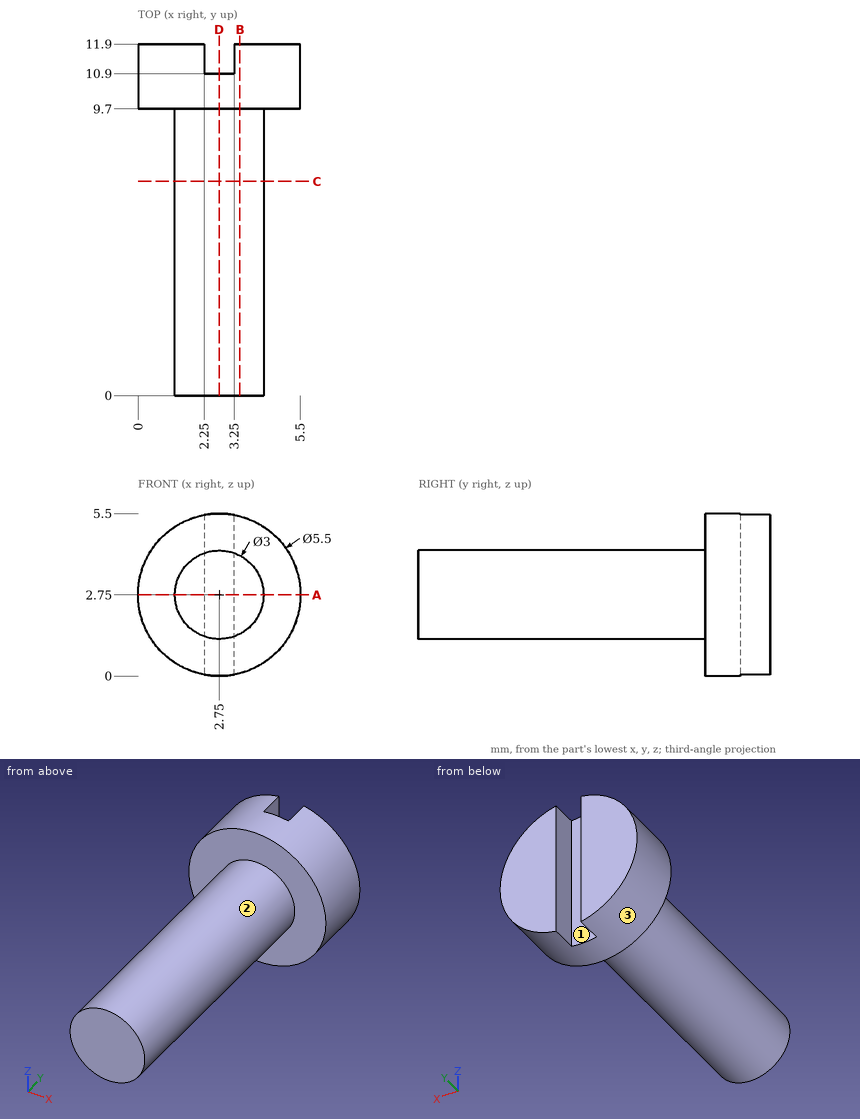
Answer from the drawing. Dimensions are ordinates in mm from the lowest x, y and z of the part. A direction names the side the tool comes from. Round coordinates to 2 decimals unless told otherwise and drop trailing zeros. Loops run counter-clockwise (first coordinate to the right, second up) from the corner with the lowest first, then second, coordinate; pieces in that order, holes last. Notation, with made-up numbers: (-5.5, 28.5) - (40.5, 28.5) arc R17 ccw to (40.5, 54.5) - close; hole circle Ø2 at (48.5, -26). An arc over 180 degrees is marked (long way). One line per item, written item: value.
Q1. For the marked faces 1, 2 and 3, determine the directions among +Z, -Z, +X, -X, +Y, -Y from which every point of the face is accessible in a straight line to the end or side of a thin tool.
Check values:
face 1: +Z, -Z, +Y
face 2: -Y
face 3: +Y, -Y
Q2. Find section C-C on y = 7.25. Give the vertices of the cut face in (x, z), and give its area (3 significant figures).
Check values:
outline: circle Ø3 at (2.75, 2.75)
area: 7.07 mm2
Q3. Find section A-A on z = 2.75. Give the vertices of the cut face in (x, y), and give its area (3 significant figures).
Check values:
outline: (0, 9.7) - (1.25, 9.7) - (1.25, 0) - (4.25, 0) - (4.25, 9.7) - (5.5, 9.7) - (5.5, 11.9) - (3.25, 11.9) - (3.25, 10.9) - (2.25, 10.9) - (2.25, 11.9) - (0, 11.9) - close
area: 40.2 mm2
Q4. Straight lines are drawn through the part: probe 1 along Y at (x, z) = (2.5, 3.2); probe 2 along Z at (x, y) = (2.8, 1.5); probe 3 along Y at (x, z) = (3.55, 1.3). For each, find the intervals that lie inside material, in ascending order.
Check values:
probe 1: 0 to 10.9
probe 2: 1.25 to 4.25
probe 3: 9.7 to 11.9
Q5. Each of these flat-tipped pins is pushed along its axis until it touches: pin 1 Ø2 at (x, y) = (1, 10.5) entering from -Z; pin 2 Ø0.8 at (y, z) = (11.5, 2) entering from -X; pin 3 Ø2 at (x, y) = (1, 8) entering from +Z. Where does it stop, or does it pass through?
Check values:
pin 1: z = 0.1
pin 2: x = 0.02
pin 3: z = 4.05
Q6. Find section D-D on x = 2.75. Give the vertices of the cut face in (y, z).
Check values:
outline: (0, 1.25) - (9.7, 1.25) - (9.7, 0) - (10.9, 0) - (10.9, 5.5) - (9.7, 5.5) - (9.7, 4.25) - (0, 4.25) - close
Q7. Find section B-B on x = 3.45. Give the vertices of the cut face in (y, z).
Check values:
outline: (0, 1.42) - (9.7, 1.42) - (9.7, 0.09) - (11.9, 0.09) - (11.9, 5.41) - (9.7, 5.41) - (9.7, 4.08) - (0, 4.08) - close
